The drawing under review shows one solid part. Ordinate dimensions are in mm from its lowest x, y, z. Round coordinates to 2 decimals unless told otherwise and drop trailing zeros. Order: outer loops, then holes, each group sorted by start corner. A loop starts at its lowest first (then second) coordinate and runs counter-clockwise, first axis right, second up. Notation, with made-up numbers: M 63.25,42 L 109.25,42 A30 cw 109.25,73 Z; hole C 27,-27.5 d1. An arc over 180 degrees is marked long. Answer as a JSON object with one key per item and string values.
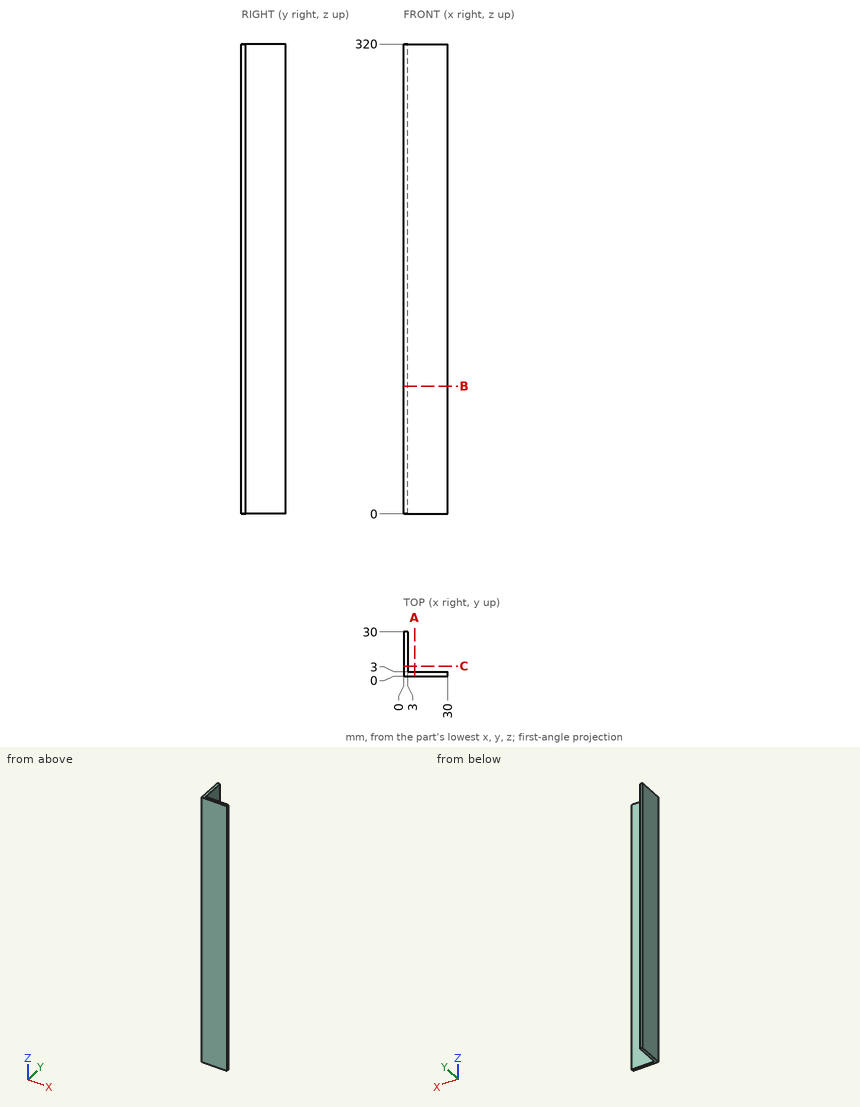
1) Add section A-A on x = 7.5. State the section outline as (y, z) points.
Geometry check:
{"outline": "M 0,0 L 3,0 L 3,320 L 0,320 Z"}
2) For L1, parallel to Y at x = 16.25, z = 155.5, list the stretches that pass through material, from the lowest coordinate up.
Geometry check:
{"L1": "y = 0 to 3"}
3) Insertion check: P1, Ø4, axis at x = 11.5, z = 171, coming from the +Y side. The pin has a flat end and moves straight along its axis. Give the tip position at first contact, or say it passes through.
Geometry check:
{"P1": "stops at y = 3"}
4) Add section B-B on z = 87. State the section outline as (x, y) points.
Geometry check:
{"outline": "M 0,0 L 30,0 L 30,3 L 3,3 L 3,30 L 0,30 Z"}
